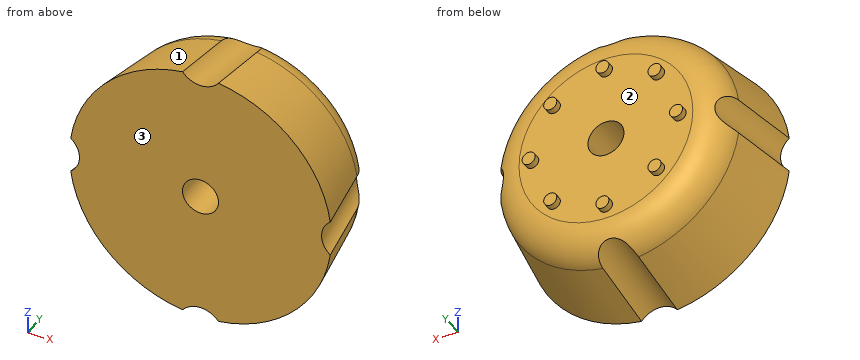
from build123d import *

# Parameters (mm, degrees)
F2_R     = 0.4
F3_DEPTH = 0.4
F6_COUNT = 4
F8_R     = 1.1
F9_DEPTH = 6.001


with BuildPart() as f1:
    # F0 (on Top) → F1 (revolve)
    with BuildSketch(Plane.XY):
        with BuildLine():
            Line((-8, 0), (0, 0))
            Line((0, 0), (0, 6))
            Line((0, 6), (-5.305746, 6))
            ThreePointArc((-5.305746, 6), (-6.598496, 5.52604), (-7.278534, 4.328798))
            Line((-7.278534, 4.328798), (-8, 0))
        make_face()
    revolve(axis=Axis((0, 13.402597, 0), (0, 1, 0)))

    # F2 (on face) → F3 (join)
    with BuildSketch(Plane(origin=(0, 6, 0), x_dir=(-1, 0, 0), z_dir=(0, 1, 0))):
        with Locations((0, 4.5)):
            Circle(F2_R)
        with Locations((4.5, 0)):
            Circle(F2_R)
        with Locations((0, -4.5)):
            Circle(F2_R)
        with Locations((-4.5, 0)):
            Circle(F2_R)
        with Locations((-3.181981, 3.181981)):
            Circle(F2_R)
        with Locations((3.181981, 3.181981)):
            Circle(F2_R)
        with Locations((3.181981, -3.181981)):
            Circle(F2_R)
        with Locations((-3.181981, -3.181981)):
            Circle(F2_R)
    extrude(amount=F3_DEPTH)


with BuildPart() as f5:
    # F4 (on Right) → F5 (revolve)
    with BuildSketch(Plane.YZ):
        Polygon((-0.443557, 10.304272), (-0.673715, 8.923321), (6.578678, 7.714589), (6.808836, 9.09554), align=None)
    revolve(axis=Axis((0, 5.520192, 7.891003), (0, 0.986394, -0.164399)))


with BuildPart() as f6_1:
    # F6: instance of F5
    add(f5.part.rotate(Axis((0, 0, 0), (0, 1, 0)), 1 * 360 / F6_COUNT))


with BuildPart() as f6_2:
    # F6: instance of F5
    add(f5.part.rotate(Axis((0, 0, 0), (0, 1, 0)), 2 * 360 / F6_COUNT))


with BuildPart() as f6_3:
    # F6: instance of F5
    add(f5.part.rotate(Axis((0, 0, 0), (0, 1, 0)), 3 * 360 / F6_COUNT))


with BuildPart() as f1_1:
    add(f1.part)

    # F7: cut F5, F6_1, F6_2, F6_3
    add(f5.part, mode=Mode.SUBTRACT)
    add(f6_1.part, mode=Mode.SUBTRACT)
    add(f6_2.part, mode=Mode.SUBTRACT)
    add(f6_3.part, mode=Mode.SUBTRACT)

    # F8 (on face) → F9 (cut, through all)
    with BuildSketch(Plane(origin=(0, 6, 0), x_dir=(-1, 0, 0), z_dir=(0, 1, 0))):
        Circle(F8_R)
    extrude(amount=-F9_DEPTH, mode=Mode.SUBTRACT)


solid = f1_1.part
Verification items for the finished model (mm, model axes). Face numbers are marked on the shaded views. Give positions to 0.01 mm unless a question says otherwise; leave off trailing zeros. Order: outer loops, then holes, each group sorted by start corner. A loop starts at its lowest first (then second) coordinate and runs counter-clockwise, first axis right, second up. Notation, with made-up numbers: M -11,-23 L 20,-23 A21 ccw 20,-11 Z; hole C 68.5,72 d7. An arc over 180 degrees is marked long. Use one line per item in the form item = value. Start each with the question number.
Q1. Scan lines: line 1 along Y through (x, z) = (2.25, -1.5); line 2 along Z through (x, y) = (-0.25, 1); line 3 along Y through (x, z) = (6, -1.25). Record each from-to range of solid material in increasing order. Write a range as [from, to].
Q2. Section check A-A (x = 0). Enter the section's corners in (y, z), then the cut area to 3 significant figures.
Q3. Go/stop test with flat-tipped pins: pin 1 Ø2.5 at (x, z) = (0, 0) entering from +Y; pin 2 Ø1.5 at (y, z) = (1.5, 5) entering from -X. Record where each tip stops, or that it passes through.
Q4. Mould release check, pull along X, two halves, no side actions. Record for the marked faces 1, 2 and 3: +X half, -X half, draft (parallel to the pull), parting line (faces both ways), or undercut.
Evaluation:
q1.line_1 = [0, 6]
q1.line_2 = [-7.25, -1.07], [1.07, 7.25]
q1.line_3 = [0, 5.82]
q2.outline = M 0,-7.39 L 5.64,-6.45 A2 ccw 6,-5.31 L 6,-4.9 L 6.4,-4.9 L 6.4,-4.1 L 6,-4.1 L 6,-1.1 L 0,-1.1 Z; M 0,1.1 L 6,1.1 L 6,4.1 L 6.4,4.1 L 6.4,4.9 L 6,4.9 L 6,5.31 A2 ccw 5.64,6.45 L 0,7.39 Z
q2.area = 69.9 mm2
q3.pin_1 = 6
q3.pin_2 = -6.5
q4.face_1 = -X half
q4.face_2 = undercut
q4.face_3 = draft
